Could you check a few things on this model? Use its own coordinates, in mm. A direction names the side the tool comes from. Round coordinates to 2 decimals unless told otherwise and drop trailing zeros. Loops run counter-clockwise (first coordinate to the right, second up) from the corner with the lowest first, then second, coordinate; pieces in that order, holes last. Notation, with made-up numbers: (83.25, -32) -> (107.25, -32) arc R30 ccw to (107.25, -3) -> close; hole circle Ø3 at (-19.75, 78). An arc over 180 degrees is marked (long way). Write each question's results on one line, items separated by ' | '.
Autodesk Inventor part; units mm, degrees
ref_plane "YZ Plane" through (0, 0, 0) normal (1, 0, 0) x (0, 1, 0)
ref_plane "XZ Plane" through (0, 0, 0) normal (0, 1, 0) x (-1, 0, 0)
ref_plane "XY Plane" through (0, 0, 0) normal (0, 0, 1) x (1, 0, 0)
sketch "Sketch2" plane through (0, 0, 0) normal (0, 1, 0) x (-1, 0, 0)
  line L0 (-50.8, 50.8) -> (50.8, 50.8)
  line L1 (57.15, 44.45) -> (57.15, -44.45)
  line L2 (50.8, -50.8) -> (-50.8, -50.8)
  line L3 (-57.15, -44.45) -> (-57.15, 44.45)
  arc A0 (-50.8, 50.8) -> (-57.15, 44.45) centre (-50.8, 44.45) ccw
  arc A1 (-57.15, -44.45) -> (-50.8, -50.8) centre (-50.8, -44.45) ccw
  arc A2 (50.8, -50.8) -> (57.15, -44.45) centre (50.8, -44.45) ccw
  arc A3 (57.15, 44.45) -> (50.8, 50.8) centre (50.8, 44.45) ccw
  line L4 (50.8, 48.768) -> (-50.8, 48.768)
  arc A4 (-50.8, 48.768) -> (-55.118, 44.45) centre (-50.8, 44.45) ccw
  line L5 (-55.118, 44.45) -> (-55.118, -44.45)
  arc A5 (-55.118, -44.45) -> (-50.8, -48.768) centre (-50.8, -44.45) ccw
  line L6 (-50.8, -48.768) -> (50.8, -48.768)
  arc A6 (50.8, -48.768) -> (55.118, -44.45) centre (50.8, -44.45) ccw
  line L7 (55.118, -44.45) -> (55.118, 44.45)
  arc A7 (55.118, 44.45) -> (50.8, 48.768) centre (50.8, 44.45) ccw
  line L8 (-50.8, 44.45) -> (50.8, -44.45) construction
  point P0 (0, 0)
  point P1 (0, 0)
  point P2 (0, 0)
  dimension "d0" = 114.3
  dimension "d1" = 101.6
  dimension "d2" = 6.35
  dimension "d3" = 2.032
extrude "Extrusion1" add sketch "Sketch2" along normal blind 4.572
sketch "Sketch3" plane through (0, 4.572, 0) normal (0, 1, 0) x (1, 0, 0)
  line L0 (-55.118, -44.45) -> (-55.118, 44.45)
  arc A0 (-50.8, 48.768) -> (-55.118, 44.45) centre (-50.8, 44.45) ccw
  line L1 (-50.8, 48.768) -> (50.8, 48.768)
  line L2 (55.118, 44.45) -> (55.118, -44.45)
  line L3 (50.8, -48.768) -> (-50.8, -48.768)
  line L4 (-50.8, 49.784) -> (50.8, 49.784)
  line L5 (56.134, 44.45) -> (56.134, -44.45)
  line L6 (50.8, -49.784) -> (-50.8, -49.784)
  line L7 (-56.134, -44.45) -> (-56.134, 44.45)
  arc A1 (-50.8, 49.784) -> (-56.134, 44.45) centre (-50.8, 44.45) ccw
  arc A2 (-56.134, -44.45) -> (-50.8, -49.784) centre (-50.8, -44.45) ccw
  arc A3 (50.8, -49.784) -> (56.134, -44.45) centre (50.8, -44.45) ccw
  arc A4 (56.134, 44.45) -> (50.8, 49.784) centre (50.8, 44.45) ccw
  line L8 (-54.102, 44.45) -> (-54.102, -44.45)
  arc A5 (-54.102, -44.45) -> (-50.8, -47.752) centre (-50.8, -44.45) ccw
  line L9 (-50.8, -47.752) -> (50.8, -47.752)
  arc A6 (50.8, -47.752) -> (54.102, -44.45) centre (50.8, -44.45) ccw
  line L10 (54.102, -44.45) -> (54.102, 44.45)
  arc A7 (54.102, 44.45) -> (50.8, 47.752) centre (50.8, 44.45) ccw
  line L11 (50.8, 47.752) -> (-50.8, 47.752)
  arc A8 (-50.8, 47.752) -> (-54.102, 44.45) centre (-50.8, 44.45) ccw
  point P0 (0, 0)
  dimension "d7" = 1.016
  dimension "d8" = 1.016
  dimension "d9" = 1.016
  dimension "d10" = 1.016
  dimension "d11" = 2.032
extrude "Extrusion2" add sketch "Sketch3" along normal blind 10.16
sketch "Sketch5" plane through (0, 14.732, 0) normal (0, 1, 0) x (1, 0, 0)
  arc A0 (-50.8, 49.784) -> (-56.134, 44.45) centre (-50.8, 44.45) ccw
  line L0 (-56.134, -44.45) -> (-56.134, 44.45)
  arc A1 (-56.134, -44.45) -> (-50.8, -49.784) centre (-50.8, -44.45) ccw
  line L1 (50.8, -49.784) -> (-50.8, -49.784)
  arc A2 (50.8, -49.784) -> (56.134, -44.45) centre (50.8, -44.45) ccw
  line L2 (56.134, 44.45) -> (56.134, -44.45)
  arc A3 (56.134, 44.45) -> (50.8, 49.784) centre (50.8, 44.45) ccw
  line L3 (-50.8, 49.784) -> (50.8, 49.784)
  point P0 (0, 0)
extrude "Extrusion3" add sketch "Sketch5" along normal blind 3.048
sketch "Sketch6" plane through (0, 17.78, 0) normal (0, 1, 0) x (1, 0, 0)
  line L0 (-50.8, 49.784) -> (50.8, 49.784)
  line L1 (-56.134, -44.45) -> (-56.134, 44.45)
  line L2 (56.134, 44.45) -> (56.134, -44.45)
  circle A0 centre (-46.736, 40.386) radius 2.921
  circle A1 centre (-46.736, -40.386) radius 2.921
  circle A2 centre (46.736, -40.386) radius 2.921
  circle A3 centre (46.736, 40.386) radius 2.921
  line L3 (-46.736, 40.386) -> (-46.736, -40.386) construction
  line L4 (-46.736, -40.386) -> (46.736, -40.386) construction
  line L5 (46.736, -40.386) -> (46.736, 40.386) construction
  line L6 (46.736, 40.386) -> (-46.736, 40.386) construction
  line L7 (-46.736, 40.386) -> (46.736, -40.386) construction
  point P0 (0, 0)
  point P1 (0, 0)
  dimension "d16" = 5.842
  dimension "d20" = 87.63
  dimension "d21" = 9.398
  dimension "d22" = 9.398
extrude "Extrusion4" cut sketch "Sketch6" against normal through all
properties part number "Plate"
1) I want a section at C-C, the plane x = -48. Write out the boundary of the cut face in (y, z), plus the area to 3 significant figures.
Model answer:
outline: (0, -50.8) -> (4.57, -50.8) -> (4.57, -49.78) -> (17.78, -49.78) -> (17.78, -43.02) -> (14.73, -43.02) -> (14.73, -47.75) -> (4.57, -47.75) -> (4.57, -48.77) -> (0, -48.77) -> close; (0, 48.77) -> (4.57, 48.77) -> (4.57, 47.75) -> (14.73, 47.75) -> (14.73, 43.02) -> (17.78, 43.02) -> (17.78, 49.78) -> (4.57, 49.78) -> (4.57, 50.8) -> (0, 50.8) -> close; (14.73, -37.75) -> (17.78, -37.75) -> (17.78, 37.75) -> (14.73, 37.75) -> close | area: 331 mm2
2) I want a section at B-B, the plane z = 9. Write out the boundary of the cut face in (x, y).
Model answer:
outline: (-57.15, 0) -> (-55.12, 0) -> (-55.12, 4.57) -> (-54.1, 4.57) -> (-54.1, 14.73) -> (54.1, 14.73) -> (54.1, 4.57) -> (55.12, 4.57) -> (55.12, 0) -> (57.15, 0) -> (57.15, 4.57) -> (56.13, 4.57) -> (56.13, 17.78) -> (-56.13, 17.78) -> (-56.13, 4.57) -> (-57.15, 4.57) -> close
3) I want a section at A-A, the plane y = 2.75. Write out the boundary of the cut face in (x, z), plus the area to 3 significant figures.
Model answer:
outline: (-57.15, -44.45) arc R6.35 ccw to (-50.8, -50.8) -> (50.8, -50.8) arc R6.35 ccw to (57.15, -44.45) -> (57.15, 44.45) arc R6.35 ccw to (50.8, 50.8) -> (-50.8, 50.8) arc R6.35 ccw to (-57.15, 44.45) -> close; hole (-55.12, -44.45) arc R4.32 ccw to (-50.8, -48.77) -> (50.8, -48.77) arc R4.32 ccw to (55.12, -44.45) -> (55.12, 44.45) arc R4.32 ccw to (50.8, 48.77) -> (-50.8, 48.77) arc R4.32 ccw to (-55.12, 44.45) -> close | area: 842 mm2
4) If we mould it in two halves opening along Z, with no side actions, what happens to faces 1 (the flat face through (-54.102, 10, -1)), 2 (the flat face through (-57.15, 2, 1)), 3 (the cylindrical face through (-54.53, 11.084, 48.263))? For each: released by +Z, released by -Z, zero draft, split by the parting line, or undercut.
Model answer:
face 1: undercut | face 2: zero draft | face 3: released by +Z
5) I'm going to push flat-ended pins straight in: pin 1 (9.5 mm diameter, centred on x = -46.736, z = 40.386, fed in from +Y); pin 2 (4 mm diameter, centred on y = 10.5, z = 10.5, fed in from +X); pin 3 (3 mm diameter, centred on x = -10.5, z = 19, fed in from -Y); pin 4 (6.5 mm diameter, centred on x = 7, y = 10.5, fed in from +Z). Where does each tip first touch, or does it pass through?
Model answer:
pin 1: stops at y = 17.78 | pin 2: stops at x = 56.13 | pin 3: stops at y = 14.73 | pin 4: stops at z = 49.78
6) I need wall thicknesses on line 1 (X direction, y = 9.5, z = 4); line 2 (Z direction, x = -30.5, y = 10.75); line 3 (Z direction, x = 13.5, y = 15). Which ranges of each line are inside material? Lowest first, please.
Model answer:
line 1: x = -56.13 to -54.1, 54.1 to 56.13 | line 2: z = -49.78 to -47.75, 47.75 to 49.78 | line 3: z = -49.78 to 49.78
7) I want a section at D-D, the plane x = 39. Write out the boundary of the cut face in (y, z), plus the area to 3 significant figures.
Model answer:
outline: (0, -50.8) -> (4.57, -50.8) -> (4.57, -49.78) -> (17.78, -49.78) -> (17.78, 49.78) -> (4.57, 49.78) -> (4.57, 50.8) -> (0, 50.8) -> (0, 48.77) -> (4.57, 48.77) -> (4.57, 47.75) -> (14.73, 47.75) -> (14.73, -47.75) -> (4.57, -47.75) -> (4.57, -48.77) -> (0, -48.77) -> close | area: 363 mm2
8) For faces 4 (the cylindrical face through (54.613, 11.084, 48.18)), 5 (the flat face through (1, 10, -47.752)), 6 (the flat face through (1, 11, 49.784)), 7 (the cylindrical face through (-54.613, 11.084, -48.18)), which set-ups out of +Z, -Z, +X, -X, +Y, -Y let a thin tool reach every point of the face, with its end or its side?
Model answer:
face 4: +Z, +X, +Y | face 5: -Y | face 6: +Z, +X, -X, +Y | face 7: -Z, -X, +Y
